Geometry check sheet. Reference: the model listing, model coordinates, mm. Face numbers are marked on the shaded views. Give positions to 0.01 mm unless a question says otherwise; leave off trailing zeros. Use a Markdown table: item, result. Add a question column.
from build123d import *

# Parameters (mm, degrees)
SKETCH1_R           = 32.5
SKETCH1_R_2         = 2
BOSS_EXTRUDE1_DEPTH = 28
FILLET1_R           = 10
CUT_EXTRUDE2_DEPTH  = 28


with BuildPart() as part:
    # Sketch1 → Boss-Extrude1 (new body)
    with BuildSketch(Plane(origin=(0, 0, 0), x_dir=(1, 0, 0), z_dir=(0, 1, 0))):
        with Locations(Location((0, 0, 0), (0, 0, 270))):
            Circle(SKETCH1_R)
        with Locations(Location((0, 0, 0), (0, 0, 270))):
            Circle(SKETCH1_R_2, mode=Mode.SUBTRACT)
    extrude(amount=BOSS_EXTRUDE1_DEPTH)

    # Fillet1
    fillet1_edges = [part.edges().sort_by_distance(p)[0] for p in [
        (0, 0, -32.5),
        (0, 28, -32.5),
    ]]
    fillet(fillet1_edges, radius=FILLET1_R)

    # Sketch2 → Cut-Extrude2 (cut)
    with BuildSketch(Plane(origin=(0, 28, 0), x_dir=(1, 0, 0), z_dir=(0, 1, 0))):
        with BuildLine():
            ThreePointArc((-2.72799344, 2.925414806), (-2.030153452, 3.446516642), (-1.236067977, 3.804226065))
            Line((-1.236067977, 3.804226065), (-6.180339887, 19.021130326))
            ThreePointArc((-6.180339887, 19.021130326), (-10.150767259, 17.232583209), (-13.639967201, 14.627074032))
            Line((-13.639967201, 14.627074032), (-2.72799344, 2.925414806))
        make_face()
        with BuildLine():
            ThreePointArc((2.72799344, -2.925414806), (2.030153452, -3.446516642), (1.236067977, -3.804226065))
            Line((1.236067977, -3.804226065), (6.180339887, -19.021130326))
            ThreePointArc((6.180339887, -19.021130326), (10.150767259, -17.232583209), (13.639967201, -14.627074032))
            Line((13.639967201, -14.627074032), (2.72799344, -2.925414806))
        make_face()
        with BuildLine():
            ThreePointArc((0.487477374, -3.970184607), (-0.38338301, -3.981584793), (-1.236067977, -3.804226065))
            Line((-1.236067977, -3.804226065), (-6.180339887, -19.021130326))
            ThreePointArc((-6.180339887, -19.021130326), (-1.91691505, -19.907923967), (2.437386868, -19.850923033))
            Line((2.437386868, -19.850923033), (0.487477374, -3.970184607))
        make_face()
        with BuildLine():
            ThreePointArc((-0.487477374, 3.970184607), (0.38338301, 3.981584793), (1.236067977, 3.804226065))
            Line((1.236067977, 3.804226065), (6.180339887, 19.021130326))
            ThreePointArc((6.180339887, 19.021130326), (1.91691505, 19.907923967), (-2.437386868, 19.850923033))
            Line((-2.437386868, 19.850923033), (-0.487477374, 3.970184607))
        make_face()
        with BuildLine():
            ThreePointArc((1.939238481, 3.498478829), (2.650480193, 2.995822883), (3.236067977, 2.351141009))
            Line((3.236067977, 2.351141009), (16.180339887, 11.755705046))
            ThreePointArc((16.180339887, 11.755705046), (13.252400964, 14.979114416), (9.696192405, 17.492394143))
            Line((9.696192405, 17.492394143), (1.939238481, 3.498478829))
        make_face()
        with BuildLine():
            ThreePointArc((-1.939238481, -3.498478829), (-2.650480193, -2.995822883), (-3.236067977, -2.351141009))
            Line((-3.236067977, -2.351141009), (-16.180339887, -11.755705046))
            ThreePointArc((-16.180339887, -11.755705046), (-13.252400964, -14.979114416), (-9.696192405, -17.492394143))
            Line((-9.696192405, -17.492394143), (-1.939238481, -3.498478829))
        make_face()
        with BuildLine():
            ThreePointArc((3.625231148, 1.690473047), (3.905184028, 0.865758456), (4, 0))
            Line((4, 0), (20, 0))
            ThreePointArc((20, 0), (19.525920142, 4.328792279), (18.126155741, 8.452365235))
            Line((18.126155741, 8.452365235), (3.625231148, 1.690473047))
        make_face()
        with BuildLine():
            ThreePointArc((-3.625231148, -1.690473047), (-3.905184028, -0.865758456), (-4, 0))
            Line((-4, 0), (-20, 0))
            ThreePointArc((-20, 0), (-19.525920142, -4.328792279), (-18.126155741, -8.452365235))
            Line((-18.126155741, -8.452365235), (-3.625231148, -1.690473047))
        make_face()
        with BuildLine():
            Line((19.632543669, -3.816179908), (3.926508734, -0.763235982))
            ThreePointArc((3.926508734, -0.763235982), (3.668240298, -1.594996276), (3.236067977, -2.351141009))
            Line((3.236067977, -2.351141009), (16.180339887, -11.755705046))
            ThreePointArc((16.180339887, -11.755705046), (18.341201488, -7.974981379), (19.632543669, -3.816179908))
        make_face()
        with BuildLine():
            ThreePointArc((-3.926508734, 0.763235982), (-3.668240298, 1.594996276), (-3.236067977, 2.351141009))
            Line((-3.236067977, 2.351141009), (-16.180339887, 11.755705046))
            ThreePointArc((-16.180339887, 11.755705046), (-18.341201488, 7.974981379), (-19.632543669, 3.816179908))
            Line((-19.632543669, 3.816179908), (-3.926508734, 0.763235982))
        make_face()
    extrude(amount=-CUT_EXTRUDE2_DEPTH, mode=Mode.SUBTRACT)


solid = part.part
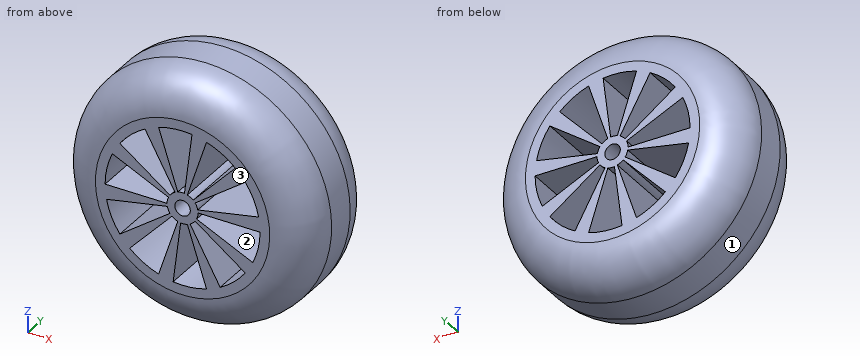
1) Gauge pin test, flat ends, axial feed: P1, Ø1.5, axis at x = -4, y = 3, coming from the +Z side; P2, Ø12, axis at y = 6, z = -24.5, coming from the -X side; P3, Ø2, axis at x = 2.5, y = 23, coming from the -Z side. Record the tip position at first contact, or that the pin passes through.
2) Material ranges on probe 1 along Z at (x, y) = (-12, 10.5); probe 2 along Z at (x, y) = (6.5, 13); probe 3 along X at (y, z) = (1.75, -12), recorded low to high. Write a range as [from, to].
3) Sectioned sample at A-A, the plane y = 2. Count the separate pieces of the cut face and the enclosed holes in it, and give its area (3 significant figures).
4) Draft check along Z on the marked faces 1, 2 and 3. Enter one of: +Z half, -Z half, draft (parallel to the pull), parting line (faces both ways), or undercut.
Check values:
| question | item | result |
|---|---|---|
| 1 | P1 | z = 30.05 |
| 1 | P2 | x = -26.23 |
| 1 | P3 | z = -31.57 |
| 2 | probe 1 | [-30.2, -16], [-12.87, -8.72], [-2.33, 0], [5.6, 8.72], [16, 30.2] |
| 2 | probe 2 | [-31.84, -11.73], [-4.72, -3.03], [0, 1.26], [4.72, 6.97], [18.91, 31.84] |
| 2 | probe 3 | [-25.47, -11.19], [-3.9, -1.47], [3.9, 6.65], [16, 25.47] |
| 3 | separate pieces | 1 |
| 3 | enclosed holes | 11 |
| 3 | area | 1,700 mm² |
| 4 | face 1 | parting line |
| 4 | face 2 | undercut |
| 4 | face 3 | draft |
